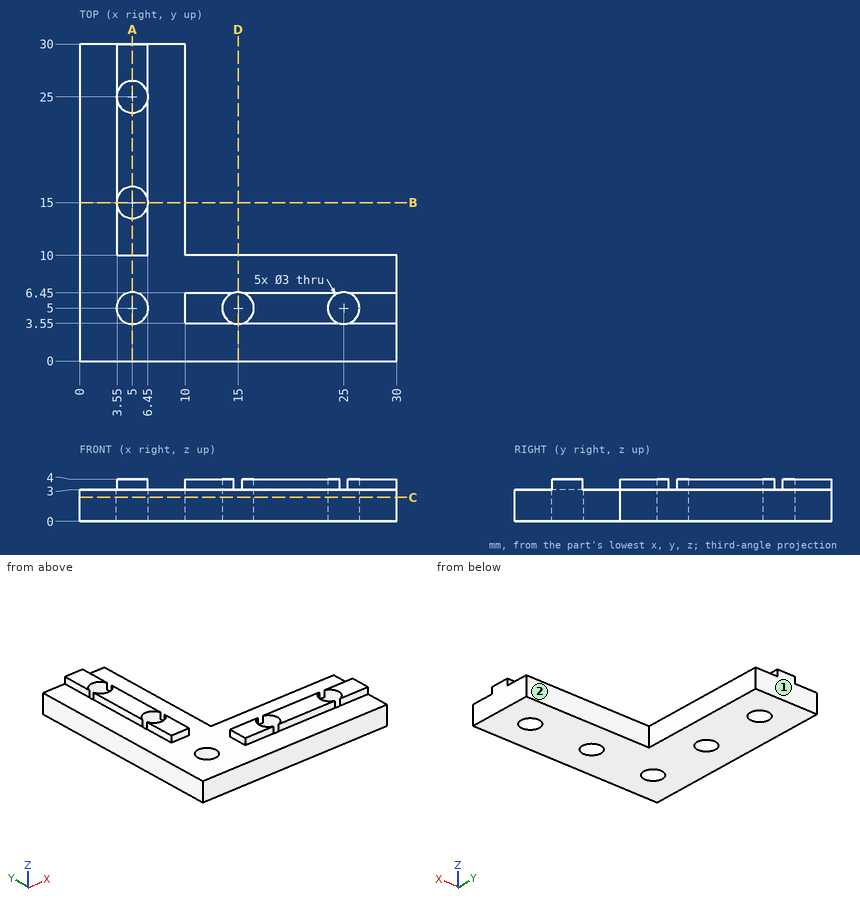
Source: three-view drawing plus pictorial views. Frame: mm from the lowest corner of the part. A direction names the side the tool comes from. Coordinates: 2 decimals unless noted, no trailing zeros. Order: outer loops, then holes, each group sorted by start corner. A loop starts at its lowest first (then second) coordinate and runs counter-clockwise, first axis right, second up. Notation, with made-up numbers: M 59,63.25 L 97,63.25 A19 ccw 97,86.25 Z; hole C 49,20 d10. An arc over 180 degrees is marked long. Write each question's results on one line, items separated by ' | '. Start each with the question number.
1. Pin query (flat end, axial travel): pin 1 (0.8 mm diameter, centred on x = 12, z = 3.5, fed in from +Y); pin 2 (2 mm diameter, centred on x = 13, z = 1.5, fed in from +Y); pin 3 (0.5 mm diameter, centred on y = 21, z = 3.5, fed in from -X). Return the tip coordinate at first contact, or that it passes through.
2. Section A-A, the plane x = 5. Return the cut outline in (y, z), then the cut area to 3 significant figures.
3. Section B-B, the plane y = 15. Return the cut outline in (x, z).
4. Section C-C, the plane z = 2.25. Return the cut outline in (x, y).
5. Material intervals for L1, parallel to Y at x = 5, z = 2.8; L2, parallel to Y at x = 15, z = 2.75; L3, parallel to X at y = 4.75, z = 1.45, sorted ascending.
6. Reachability of the marked faces 1 and 2 from +Z, -Z, +X, -X, +Y, -Y: full face, straight path, thin tool, end or side. Return the list, or none.
Solution:
1) pin 1: y = 6.45 | pin 2: y = 10 | pin 3: x = 3.55
2) outline: M 0,0 L 3.5,0 L 3.5,3 L 0,3 Z; M 6.5,0 L 13.5,0 L 13.5,4 L 10,4 L 10,3 L 6.5,3 Z; M 16.5,0 L 23.5,0 L 23.5,4 L 16.5,4 Z; M 26.5,0 L 30,0 L 30,4 L 26.5,4 Z | area: 77.0 mm²
3) outline: M 0,0 L 3.5,0 L 3.5,3 L 0,3 Z; M 6.5,0 L 10,0 L 10,3 L 6.5,3 Z
4) outline: M 0,0 L 30,0 L 30,10 L 10,10 L 10,30 L 0,30 Z; hole C 5,5 d3; hole C 5,15 d3; hole C 5,25 d3; hole C 15,5 d3; hole C 25,5 d3
5) L1: 0 to 3.5, 6.5 to 13.5, 16.5 to 23.5, 26.5 to 30 | L2: 0 to 3.5, 6.5 to 10 | L3: 0 to 3.52, 6.48 to 13.52, 16.48 to 23.52, 26.48 to 30
6) face 1: +Z, -Z, +X, -X, +Y | face 2: +Z, -Z, +X, +Y
